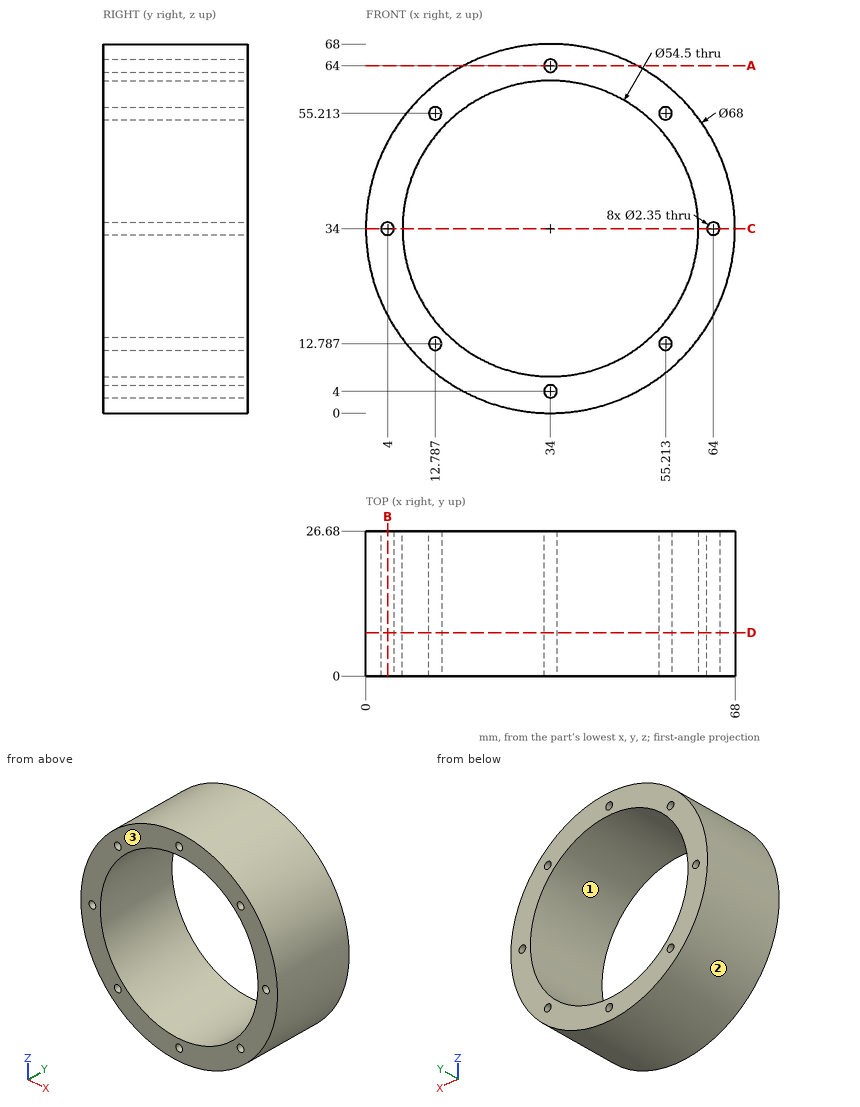
The figure shows three views and two pictorial views of one solid part (mm, origin at its lowest corner). Answer the questions. Give positions to 0.01 mm unless a question says otherwise; leave off trailing zeros. Write each loop counter-clockwise with the first axis right and the second up, starting at its lowest first coordinate (ties: lowest second). Pieces come first, ordered by that corner, then holes. Notation, with made-up numbers: M -40,76 L -8,76 A27 cw -8,96 Z; hole C 31.5,-6 d4. An arc over 180 degrees is marked long. One line per item, written item: value. Start each with the question number.
(1) Determine the mould class of the marked faces 1, 2 and 3 for opening direction X: pulls with the +X half, pulls with the -X half, needs draft (parallel to the pull), parting line crosses it, or undercut.
(2) Find section B-B (x = 4). Determine the outline of the cut face in (y, z) (3 decimals).
(3) Find the intervals of material crossed by line 1 (Z direction, x = 34, y = 10) (3 decimals); line 2 (X direction, y = 19, z = 55) (1 decimal); line 3 (Z direction, x = 14.5, y = 20.75) (1 decimal), in increasing order.
(4) Find section C-C (z = 34). Determine the outline of the cut face in (x, y) (3 decimals), plus the area to 3 significant figures.
(5) Find section D-D (y = 8). Give the number of separate pieces and of enclosed holes in the cut face, plus the area to 3 significant figures.
(6) Flat-ended cylindrical pins translate along their axes: pin 1 Ø8 at (x, y) = (19.5, 5) entering from -Z; pin 2 Ø1.9 at (x, z) = (55.21, 55.21) entering from +Y; pin 3 Ø1.5 at (x, y) = (50.5, 18.5) entering from -Z; pin 4 Ø12 at (y, z) = (20, 57.5) entering from +X. Find the tip coordinate at first contact, or state that the pin passes through.
(7) Find section A-A (z = 64). Determine the outline of the cut face in (x, y) (3 decimals).
Results below:
1. face 1: undercut
1. face 2: parting line crosses it
1. face 3: needs draft
2. outline: M 0,18 L 26.68,18 L 26.68,32.825 L 0,32.825 Z; M 0,35.175 L 26.68,35.175 L 26.68,50 L 0,50 Z
3. line 1: z = 0 to 2.825, 5.175 to 6.75, 61.25 to 62.825, 65.175 to 68
3. line 2: x = 7.3 to 11.6, 13.9 to 16.6, 51.4 to 54.1, 56.4 to 60.7
3. line 3: z = 6.1 to 15, 53 to 61.9
4. outline: M 0,0 L 2.825,0 L 2.825,26.68 L 0,26.68 Z; M 5.175,0 L 6.75,0 L 6.75,26.68 L 5.175,26.68 Z; M 61.25,0 L 62.825,0 L 62.825,26.68 L 61.25,26.68 Z; M 65.175,0 L 68,0 L 68,26.68 L 65.175,26.68 Z
4. area: 235 mm^2
5. separate pieces: 1
5. enclosed holes: 9
5. area: 1,260 mm^2
6. pin 1: stops at z = 1.66
6. pin 2: passes through
6. pin 3: stops at z = 3.87
6. pin 4: stops at x = 63.15
7. outline: M 18,0 L 32.825,0 L 32.825,26.68 L 18,26.68 Z; M 35.175,0 L 50,0 L 50,26.68 L 35.175,26.68 Z
